```python
from build123d import *

# Parameters (mm, degrees)
SKETCH1_W           = 20
SKETCH1_H           = 24
SKETCH1_R           = 1.35
BOSS_EXTRUDE1_DEPTH = 4
SKETCH2_W           = 20
SKETCH2_H           = 8
BOSS_EXTRUDE2_DEPTH = 8
SKETCH3_R           = 8.25
BOSS_EXTRUDE3_DEPTH = 8
SKETCH4_W           = 0.35
SKETCH4_H           = 20.293623418
CUT_EXTRUDE1_DEPTH  = 8
SKETCH6_R           = 1.55
CUT_EXTRUDE2_DEPTH  = 8
FILLET1_R           = 1


with BuildPart() as part:
    # Sketch1 → Boss-Extrude1 (new body)
    with BuildSketch(Plane.XY):
        with Locations((0, -1)):
            Rectangle(SKETCH1_W, SKETCH1_H)
        with Locations((5.991996797, 6)):
            Circle(SKETCH1_R, mode=Mode.SUBTRACT)
        Circle(SKETCH1_R, mode=Mode.SUBTRACT)
        with Locations((-6.008003203, 6)):
            Circle(SKETCH1_R, mode=Mode.SUBTRACT)
    extrude(amount=BOSS_EXTRUDE1_DEPTH)

    # Sketch2 → Boss-Extrude2 (add)
    with BuildSketch(Plane.XY.offset(4)):
        with Locations((0, -9)):
            Rectangle(SKETCH2_W, SKETCH2_H)
    extrude(amount=BOSS_EXTRUDE2_DEPTH)

    # Sketch3 → Boss-Extrude3 (add)
    with BuildSketch(Plane.XZ.offset(13)):
        with BuildLine():
            Line((-4, 32.881805097), (-4, 40.881805097))
            Line((-4, 40.881805097), (4, 40.881805097))
            Line((4, 40.881805097), (4, 32.881805097))
            ThreePointArc((4, 32.881805097), (0, 7), (-4, 32.881805097))
        make_face()
        with Locations((0, 20.25)):
            Circle(SKETCH3_R, mode=Mode.SUBTRACT)
    extrude(amount=-BOSS_EXTRUDE3_DEPTH)

    # Sketch4 → Cut-Extrude1 (cut)
    with BuildSketch(Plane.XZ.offset(13)):
        with Locations((0, 38.64495544)):
            Rectangle(SKETCH4_W, SKETCH4_H)
    extrude(amount=-CUT_EXTRUDE1_DEPTH, mode=Mode.SUBTRACT)

    # Sketch6 → Cut-Extrude2 (cut)
    with BuildSketch(Plane(origin=(4, 0, 0), x_dir=(0, 0, -1), z_dir=(1, 0, 0))):
        with Locations((-36.881805097, -9)):
            Circle(SKETCH6_R)
    extrude(amount=-CUT_EXTRUDE2_DEPTH, mode=Mode.SUBTRACT)

    # Fillet1
    fillet1_edges = [part.edges().sort_by_distance(p)[0] for p in [
        (10, 11, 2),
        (0, 11, 4),
        (-10, 11, 2),
        (0, 11, 0),
        (-2.0875, -5, 40.881805097),
        (-2.0875, -13, 40.881805097),
        (2.0875, -13, 40.881805097),
        (2.0875, -5, 40.881805097),
    ]]
    fillet(fillet1_edges, radius=FILLET1_R)


solid = part.part
```
The model under review builds one solid part; all positions refer to its coordinate system, in mm. A direction names the side the tool comes from. Give positions to 0.01 mm unless a question says otherwise; leave off trailing zeros. Order: outer loops, then holes, each group sorted by start corner. A loop starts at its lowest first (then second) coordinate and runs counter-clockwise, first axis right, second up. Notation, with made-up numbers: (-14.75, 26.25) - (28.25, 26.25) arc R26 cw to (28.25, 51.25) - close; hole circle Ø10 at (89.25, -7). An arc over 180 degrees is marked (long way). Use CSV: the item, a comma, the result in double quotes. Start each with the question number.
Q1. We need section C-C, the plane y = -9. Write out the cut boundary in (x, z) (3 decimals), and give its area (3 significant figures).
Q2. Tool access review of faces 1 (the flat face through (10, -4, 3)), 2 (the flat face through (-10, -4, 3)), 3 (the flat face through (4, -9, 35)), 4 (the flat face through (-0.175, -9, 35)): name each direction out of +Z, -Z, +X, -X, +Y, -Y from which nothing blocks a thin tool from reaching the whole face with its end or side.
Q3. Clearance check with flat-ended pins moving along their axes: pin 1 Ø1.6 at (x, y) = (5.99, 6) entering from +Z; pin 2 Ø9 at (y, z) = (-6, 8.5) entering from -X; pin 3 Ø1 at (x, y) = (-6, 1) entering from -Z; pin 4 Ø3.5 at (y, z) = (-9, 36.88) entering from -X. State where each tip first meets the part, or that it passes through.
Q4. We need section A-A, the plane y = 6. Write out the cut boundary in (x, z), and give its area (3 significant figures).
Q5. The part is to be moulded in two halves that separate along Y. For faces 5 (the cylindrical face through (6.718, 7.138, 1.972)), 6 (the flat face through (-2, -9, 40.882)), 7 (the cylindrical face through (2.114, -12.715, 40.581)), say which applies: +Y half, -Y half, draft (parallel to the pull), parting line (faces both ways), or undercut.
Q6. We need section D-D, the plane z = 6.5. Write out the cut boundary in (x, y), and give its area (3 significant figures).
Q7. We need section B-B, the plane z = 34. Write out the cut boundary in (x, y) (3 decimals).
Q8. To check wall thickness, follow line 1 along Y through (x, z) = (-4, 6); line 2 along Z through (x, y) = (-0.25, -1.5); line 3 along X through (y, z) = (-9.5, 15.5). State the ranges of each line that lie inside material, in increasing order. Write a range as [from, to].
Outcome:
1,outline,"(-10, 0) - (10, 0) - (10, 11.557) arc R13.25 ccw to (4, 32.882) - (4, 35.332) - (0.175, 35.332) - (0.175, 28.498) arc R8.25 cw (long way) to (-0.175, 28.498) - (-0.175, 35.332) - (-4, 35.332) - (-4, 32.882) arc R13.25 ccw to (-10, 11.557) - close; (-4, 38.432) - (-0.175, 38.432) - (-0.175, 40.882) - (-4, 40.882) - close; (0.175, 38.432) - (4, 38.432) - (4, 40.882) - (0.175, 40.882) - close"
1,area,"538 mm^2"
2,face 1,"-Z, +X, +Y, -Y"
2,face 2,"-Z, -X, +Y, -Y"
2,face 3,"+Z, +X, +Y, -Y"
2,face 4,"+Z, +Y, -Y"
3,pin 1,"passes through"
3,pin 2,"stops at x = -11.09"
3,pin 3,"stops at z = 0"
3,pin 4,"stops at x = -4"
4,outline,"(-10, 0) - (-7.36, 0) - (-7.36, 4) - (-10, 4) - close; (-4.66, 0) - (4.64, 0) - (4.64, 4) - (-4.66, 4) - close; (7.34, 0) - (10, 0) - (10, 4) - (7.34, 4) - close"
4,area,"58.4 mm^2"
5,face 5,"undercut"
5,face 6,"draft"
5,face 7,"-Y half"
6,outline,"(-10, -13) - (10, -13) - (10, -5) - (-10, -5) - close"
6,area,"160 mm^2"
7,outline,"(-4, -13) - (-0.175, -13) - (-0.175, -5) - (-4, -5) - close; (0.175, -13) - (4, -13) - (4, -5) - (0.175, -5) - close"
8,line 1,"y = [-13, -5]"
8,line 2,"z = [0, 4]"
8,line 3,"x = [-12.37, -6.75], [6.75, 12.37]"
